from build123d import *

# Parameters (mm, degrees)
SKETCH_1_R          = 35
SKETCH_1_R_2        = 3
EXTRUDE_1_DEPTH     = 6
SKETCH_3_R          = 3
CUT_EXTRUDE_2_DEPTH = 50.859803449
SKETCH_4_R          = 2
EXTRUDE_2_DEPTH     = 22
SKETCH_7_R          = 4
EXTRUDE_3_DEPTH     = 2
CHAMFER_1_SIZE      = 1


with BuildPart() as part:
    # 草图1 → 凸台-拉伸1 (new body)
    with BuildSketch(Plane.XY):
        Circle(SKETCH_1_R)
        Circle(SKETCH_1_R_2, mode=Mode.SUBTRACT)
    extrude(amount=EXTRUDE_1_DEPTH)

    # 草图3 → 切除-拉伸2 (cut, through all)
    with BuildSketch(Plane(origin=(0, 0, 0), x_dir=(-1, 0, 0), z_dir=(0, 0, -1))):
        with Locations((-4.582105158, 17.407019053)):
            Circle(SKETCH_3_R)
        with Locations((9.068583583, 15.548658842)):
            Circle(SKETCH_3_R)
        with Locations((17.407019053, 4.582105158)):
            Circle(SKETCH_3_R)
        with Locations((15.548658842, -9.068583583)):
            Circle(SKETCH_3_R)
        with Locations((4.582105158, -17.407019053)):
            Circle(SKETCH_3_R)
        with Locations((-9.068583583, -15.548658842)):
            Circle(SKETCH_3_R)
        with Locations((-17.407019053, -4.582105158)):
            Circle(SKETCH_3_R)
        with Locations((-15.548658842, 9.068583583)):
            Circle(SKETCH_3_R)
    extrude(amount=-CUT_EXTRUDE_2_DEPTH, mode=Mode.SUBTRACT)

    # 草图4 → 凸台-拉伸2 (add)
    with BuildSketch(Plane.XY.offset(6)):
        with Locations((9.178670771, -3.968879298)):
            Circle(SKETCH_4_R)
    extrude(amount=EXTRUDE_2_DEPTH)

    # 草图7 → 凸台-拉伸3 (add)
    with BuildSketch(Plane.XY.offset(28)):
        with Locations((9.178670771, -3.968879298)):
            Circle(SKETCH_7_R)
    extrude(amount=-EXTRUDE_3_DEPTH)

    # 倒角1
    chamfer_1_edges = [part.edges().sort_by_distance(p)[0] for p in [
        (7.178670771, -3.968879298, 6),
    ]]
    chamfer(chamfer_1_edges, length=CHAMFER_1_SIZE)


solid = part.part
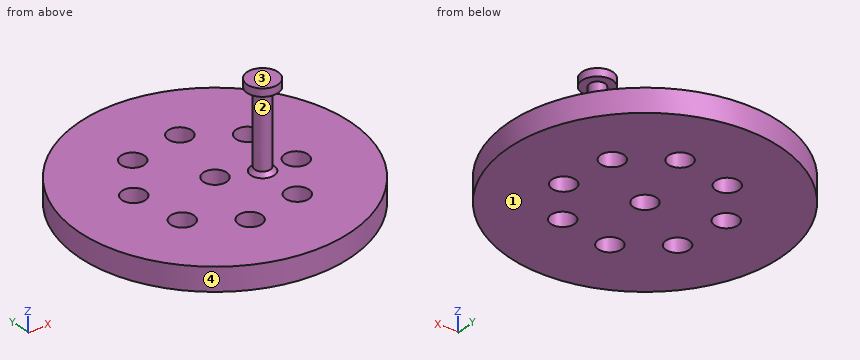
Design review of the part built by this model. Coordinates are the model's own, in mm. Face numbers are marked on the shaded views. Coordinates: 2 decimals unless noted, no trailing zeros. Loops run counter-clockwise (first coordinate to the right, second up) from the corner with the lowest first, then second, coordinate; pieces in that order, holes last. Notation, with made-up numbers: (10, 23) - (49, 23) arc R26 cw to (49, 46) - close; hole circle Ø6 at (85.5, 72.25). An arc over 180 degrees is marked (long way). Use CSV: the item, a comma, the result in double quotes. Start each with the question number.
1. Add section D-D on x = -21.5. Give the boundary of the cut face in (y, z), plus the area to 3 significant figures.
2. To check wall thickness, follow probe 1 along X at (y, z) = (2, 3.25); probe 2 along Z at (x, y) = (-9, 20.5); probe 3 along Y at (x, z) = (-20, 2). State the ranges of each line that lie inside material, in increasing order.
3. Add section A-A on x = 0. Give the boundary of the cut face in (y, z), plus the area to 3 significant figures.
4. Add section B-B on y = -19.5. Give the boundary of the cut face in (x, z), plus the area to 3 significant figures.
5. Mouldability with a two-part tool opening along Z and no side actions: class the marked faces 1, 2, 3 and 4 as released by +Z, released by -Z, zero draft, split by the parting line, or undercut.
6. Add section C-C on y = -28. Give the boundary of the cut face in (x, z).
7. Clearance check with flat-ended pins moving along their axes: pin 1 (9.5 mm diameter, centred on x = -15.55, y = -9.07, fed in from +Z); pin 2 (5.5 mm diameter, centred on x = 0, y = 0, fed in from -Z); pin 3 (12 mm diameter, centred on y = -12, z = 8.5, fed in from -X); pin 4 (12 mm diameter, centred on x = 6.5, z = 23, fed in from -Y). State where each tip first meets the part, or that it passes through.
Resolved:
1,outline,"(-27.62, 0) - (27.62, 0) - (27.62, 6) - (-27.62, 6) - close"
1,area,"331 mm2"
2,probe 1,"-34.94 to -18.93, -15.88 to -2.24, 2.24 to 34.94"
2,probe 2,"0 to 6"
2,probe 3,"-28.72 to 3.07, 6.09 to 28.72"
3,outline,"(-35, 0) - (-3, 0) - (-3, 6) - (-35, 6) - close; (3, 0) - (35, 0) - (35, 6) - (3, 6) - close"
3,area,"384 mm2"
4,outline,"(-29.06, 0) - (-6.73, 0) - (-6.73, 6) - (-29.06, 6) - close; (-2.43, 0) - (29.06, 0) - (29.06, 6) - (-2.43, 6) - close"
4,area,"323 mm2"
5,face 1,"released by -Z"
5,face 2,"undercut"
5,face 3,"released by +Z"
5,face 4,"zero draft"
6,outline,"(-21, 0) - (21, 0) - (21, 6) - (-21, 6) - close"
7,pin 1,"z = 6"
7,pin 2,"through"
7,pin 3,"x = -34.38"
7,pin 4,"y = -7.97"
